from build123d import *

# Parameters (mm, degrees)
SKETCH_2_W          = 100
SKETCH_2_H          = 40
EXTRUDE_1_DEPTH     = 150
SKETCH_3_W          = 90
SKETCH_3_H          = 32
CUT_EXTRUDE_1_DEPTH = 145
SKETCH_4_W          = 30
SKETCH_4_H          = 115
CUT_EXTRUDE_2_DEPTH = 20
SKETCH_5_W          = 35
SKETCH_5_H          = 115
CUT_EXTRUDE_3_DEPTH = 20
SKETCH_6_W          = 120
SKETCH_6_H          = 31
CUT_EXTRUDE_4_DEPTH = 207
SKETCH_7_R          = 1.5
CUT_EXTRUDE_5_DEPTH = 15
SKETCH_8_R          = 2.5
SKETCH_8_R_2        = 1.5
CUT_EXTRUDE_6_DEPTH = 15


with BuildPart() as part:
    # 草图2 → 凸台-拉伸1 (new body)
    with BuildSketch(Plane.XY):
        Rectangle(SKETCH_2_W, SKETCH_2_H)
    extrude(amount=EXTRUDE_1_DEPTH)

    # 草图3 → 切除-拉伸1 (cut)
    with BuildSketch(Plane.XY.offset(150)):
        with Locations((0.044588489, 1)):
            Rectangle(SKETCH_3_W, SKETCH_3_H)
    extrude(amount=-CUT_EXTRUDE_1_DEPTH, mode=Mode.SUBTRACT)

    # 草图4 → 切除-拉伸2 (cut)
    with BuildSketch(Plane.XZ.offset(20)):
        with Locations((-25, 77.5)):
            Rectangle(SKETCH_4_W, SKETCH_4_H)
        with Locations((25, 77.5)):
            Rectangle(SKETCH_4_W, SKETCH_4_H)
    extrude(amount=-CUT_EXTRUDE_2_DEPTH, mode=Mode.SUBTRACT)

    # 草图5 → 切除-拉伸3 (cut)
    with BuildSketch(Plane(origin=(0, 20, 0), x_dir=(1, 0, 0), z_dir=(0, 1, 0))):
        with Locations((-22.5, -77.5)):
            Rectangle(SKETCH_5_W, SKETCH_5_H)
        with Locations((22.5, -77.5)):
            Rectangle(SKETCH_5_W, SKETCH_5_H)
    extrude(amount=-CUT_EXTRUDE_3_DEPTH, mode=Mode.SUBTRACT)

    # 草图6 → 切除-拉伸4 (cut)
    with BuildSketch(Plane.ZY.offset(50)):
        with Locations((75, 0.5)):
            Rectangle(SKETCH_6_W, SKETCH_6_H)
    extrude(amount=-CUT_EXTRUDE_4_DEPTH, mode=Mode.SUBTRACT)

    # 草图7 → 切除-拉伸5 (cut)
    with BuildSketch(Plane.XZ.offset(20)):
        with Locations(Location((-5, 134, 0), (0, 0, 270))):
            Circle(SKETCH_7_R)
        with Locations(Location((5, 134, 0), (0, 0, 270))):
            Circle(SKETCH_7_R)
        with Locations(Location((5, 124, 0), (0, 0, 270))):
            Circle(SKETCH_7_R)
        with Locations(Location((-5, 124, 0), (0, 0, 270))):
            Circle(SKETCH_7_R)
    extrude(amount=-CUT_EXTRUDE_5_DEPTH, mode=Mode.SUBTRACT)

    # 草图8 → 切除-拉伸6 (cut)
    with BuildSketch(Plane.XZ.offset(20)):
        with Locations(Location((0, 129, 0), (0, 0, 270))):
            Circle(SKETCH_8_R)
        with Locations(Location((0, 74, 0), (0, 0, 270))):
            Circle(SKETCH_8_R)
        with Locations(Location((0, 19, 0), (0, 0, 270))):
            Circle(SKETCH_8_R)
        with Locations(Location((-5, 79, 0), (0, 0, 270))):
            Circle(SKETCH_8_R_2)
        with Locations(Location((-5, 69, 0), (0, 0, 270))):
            Circle(SKETCH_8_R_2)
        with Locations(Location((5, 69, 0), (0, 0, 270))):
            Circle(SKETCH_8_R_2)
        with Locations(Location((5, 79, 0), (0, 0, 270))):
            Circle(SKETCH_8_R_2)
        with Locations(Location((-5, 14, 0), (0, 0, 270))):
            Circle(SKETCH_8_R_2)
        with Locations(Location((-5, 24, 0), (0, 0, 270))):
            Circle(SKETCH_8_R_2)
        with Locations(Location((5, 24, 0), (0, 0, 270))):
            Circle(SKETCH_8_R_2)
        with Locations(Location((5, 14, 0), (0, 0, 270))):
            Circle(SKETCH_8_R_2)
    extrude(amount=-CUT_EXTRUDE_6_DEPTH, mode=Mode.SUBTRACT)


solid = part.part
Geometry check sheet. Reference: the model listing, model coordinates, mm. A direction names the side the tool comes from. Round coordinates to 2 decimals unless told otherwise and drop trailing zeros. Write each loop counter-clockwise with the first axis right and the second up, starting at its lowest first coordinate (ties: lowest second). Pieces come first, ordered by that corner, then holes. Notation, with made-up numbers: (84.25, -11.75) - (105.25, -11.75) arc R20 ccw to (105.25, -4.75) - close; hole circle Ø5 at (5.25, 65.25). An arc over 180 degrees is marked (long way). One line per item, written item: value.
1. Cross-section at D-D on z = 79. Give the number of separate pieces and of enclosed holes in the cut face, and give its area (3 significant figures).
The answers:
separate pieces: 8
enclosed holes: 0
area: 270 mm^2
2. Cross-section at B-B on z = 37.5. Record the boundary of the cut face in (x, y), and give its area (3 significant figures).
The answers:
outline: (-50, -20) - (-40, -20) - (-40, -15) - (-50, -15) - close; (-50, 16) - (-44.96, 16) - (-44.96, 17) - (-40, 17) - (-40, 20) - (-50, 20) - close; (-10, -20) - (10, -20) - (10, -15) - (-10, -15) - close; (-5, 17) - (5, 17) - (5, 20) - (-5, 20) - close; (40, -20) - (50, -20) - (50, -15) - (40, -15) - close; (40, 17) - (45.04, 17) - (45.04, 16) - (50, 16) - (50, 20) - (40, 20) - close
area: 300 mm^2
3. Set-up check for faces 1 (the face through (47, 0, 15)), 2 (the face through (-50, -18, 74)), 3 (the face through (-40, -18, 77)), 4 (the face through (5.07, -17.54, 15.5)), 5 (the face through (-1, 17, 79)): record each of +Z, -Z, +X, -X, +Y, -Y from which the full face is reachable in a straight line by a thin tool's end or side.
The answers:
face 1: +X, -X
face 2: +Z, -Z, -X, +Y, -Y
face 3: +Y, -Y
face 4: -Y
face 5: +Z
4. Depth check by flat-ended pin: pin 1 Ø1 at (x, y) = (32, -12) entering from +Z. Enter the tip coordinate at first touch or a pass-through.
The answers:
pin 1: stops at z = 5
5. Cross-section at C-C on y = 5.5. Record the boundary of the cut face in (x, z).
The answers:
outline: (-50, 0) - (50, 0) - (50, 15) - (45.04, 15) - (45.04, 5) - (-44.96, 5) - (-44.96, 15) - (-50, 15) - close; (-50, 135) - (-44.96, 135) - (-44.96, 150) - (-50, 150) - close; (45.04, 135) - (50, 135) - (50, 150) - (45.04, 150) - close
6. Cross-section at A-A on x = -16. Record the boundary of the cut face in (y, z), and give its area (3 significant figures).
The answers:
outline: (-20, 0) - (20, 0) - (20, 20) - (17, 20) - (17, 5) - (-15, 5) - (-15, 20) - (-20, 20) - close; (-20, 135) - (-15, 135) - (-15, 150) - (-20, 150) - close; (17, 135) - (20, 135) - (20, 150) - (17, 150) - close
area: 440 mm^2
7. Scan lines: L1, parallel to X at y = -17.5, z = 24; L2, parallel to X at y = -6.5, z = 138; L3, parallel to Y at x = -30.5, z = 138. Record each from-to range of solid material in increasing order.
The answers:
L1: x = -50 to -40, -10 to -6.5, -3.5 to 3.5, 6.5 to 10, 40 to 50
L2: x = -50 to -44.96, 45.04 to 50
L3: y = -20 to -15, 17 to 20
8. Mould release check, pull along Z, two halves, no side actions. Record for faces 6 (the face through (-48, 16, 74)), 7 (the face through (-4, -16, 150)), 8 (the face through (-44.955, 16.3, 88.6)): released by +Z, released by -Z, zero draft, split by the parting line, or undercut.
The answers:
face 6: undercut
face 7: released by +Z
face 8: zero draft
